```python
from build123d import *
from OCP.BRepFilletAPI import BRepFilletAPI_MakeChamfer

# Parameters (mm, degrees)
SKETCH1_W           = 8
SKETCH1_H           = 7
BOSS_EXTRUDE1_DEPTH = 17
BOSS_EXTRUDE2_DEPTH = 4
CHAMFER1_SIZE       = 2.5
CHAMFER1_SIZE_2     = 2
SKETCH3_R           = 0.4
CUT_EXTRUDE1_DEPTH  = 18.811513131
FILLET2_R           = 0.5
SKETCH4_W           = 0.5
SKETCH4_H           = 15.4
CUT_EXTRUDE2_DEPTH  = 19.814887722
SKETCH5_W           = 0.3
SKETCH5_H           = 11.5
CUT_EXTRUDE3_DEPTH  = 19.814887722
SKETCH6_R           = 0.9
CUT_EXTRUDE4_DEPTH  = 18
CHAMFER2_SIZE       = 0.5
BOSS_EXTRUDE3_START = 2
SKETCH7_R           = 2.5
SKETCH7_R_2         = 0.9
BOSS_EXTRUDE3_DEPTH = 2
BOSS_EXTRUDE4_START = 1.5
SKETCH8_R           = 0.9
SKETCH8_R_2         = 1
BOSS_EXTRUDE4_DEPTH = 1.5
BOSS_EXTRUDE5_START = 1.4
SKETCH9_R           = 1.25
SKETCH9_R_2         = 0.9
BOSS_EXTRUDE5_DEPTH = 1.4
BOSS_EXTRUDE6_START = 15
SKETCH10_R          = 2
SKETCH10_R_2        = 0.9
BOSS_EXTRUDE6_DEPTH = 15
FILLET3_R           = 0.2


# Some blends are built 0.0001 mm under size
with BuildPart() as part:
    # Sketch1 → Boss-Extrude1 (new body)
    with BuildSketch(Plane(origin=(0, 0, 0), x_dir=(1, 0, 0), z_dir=(0, 1, 0))):
        Rectangle(SKETCH1_W, SKETCH1_H)
    extrude(amount=BOSS_EXTRUDE1_DEPTH)

    # Sketch2 → Boss-Extrude2 (add)
    with BuildSketch(Plane(origin=(0, 0, 0), x_dir=(-1, 0, 0), z_dir=(0, -1, 0))):
        Polygon((-2.309401077, 0), (-1.154700538, -2), (1.154700538, -2), (2.309401077, 0), (1.154700538, 2), (-1.154700538, 2), align=None)
    extrude(amount=BOSS_EXTRUDE2_DEPTH)

    # Chamfer1
    chamfer1_edges_1 = [part.edges().sort_by_distance(p)[0] for p in [
        (1.732050808, -4, -1),
    ]]
    chamfer1_side_1 = [part.faces().sort_by_distance(p)[0] for p in [
        (1.732050808, -3.96, -1),
    ]]
    chamfer1_edges_2 = [part.edges().sort_by_distance(p)[0] for p in [
        (1.732050808, -4, 1),
    ]]
    chamfer1_side_2 = [part.faces().sort_by_distance(p)[0] for p in [
        (1.732050808, -3.96, 1),
    ]]
    chamfer1_edges_3 = [part.edges().sort_by_distance(p)[0] for p in [
        (0, -4, 2),
    ]]
    chamfer1_side_3 = [part.faces().sort_by_distance(p)[0] for p in [
        (0, -3.96, 2),
    ]]
    chamfer1_edges_4 = [part.edges().sort_by_distance(p)[0] for p in [
        (-1.732050808, -4, 1),
    ]]
    chamfer1_side_4 = [part.faces().sort_by_distance(p)[0] for p in [
        (-1.732050808, -3.96, 1),
    ]]
    chamfer1_edges_5 = [part.edges().sort_by_distance(p)[0] for p in [
        (-1.732050808, -4, -1),
    ]]
    chamfer1_side_5 = [part.faces().sort_by_distance(p)[0] for p in [
        (-1.732050808, -3.96, -1),
    ]]
    chamfer1_edges_6 = [part.edges().sort_by_distance(p)[0] for p in [
        (0, -4, -2),
    ]]
    chamfer1_side_6 = [part.faces().sort_by_distance(p)[0] for p in [
        (0, -3.96, -2),
    ]]
    chamfer1 = BRepFilletAPI_MakeChamfer(part.part.solid().wrapped)
    for e in chamfer1_edges_1:
        chamfer1.Add(CHAMFER1_SIZE - 0.0001, CHAMFER1_SIZE_2 - 0.0001, e.wrapped, chamfer1_side_1[0].wrapped)
    for e in chamfer1_edges_2:
        chamfer1.Add(CHAMFER1_SIZE - 0.0001, CHAMFER1_SIZE_2 - 0.0001, e.wrapped, chamfer1_side_2[0].wrapped)
    for e in chamfer1_edges_3:
        chamfer1.Add(CHAMFER1_SIZE - 0.0001, CHAMFER1_SIZE_2 - 0.0001, e.wrapped, chamfer1_side_3[0].wrapped)
    for e in chamfer1_edges_4:
        chamfer1.Add(CHAMFER1_SIZE - 0.0001, CHAMFER1_SIZE_2 - 0.0001, e.wrapped, chamfer1_side_4[0].wrapped)
    for e in chamfer1_edges_5:
        chamfer1.Add(CHAMFER1_SIZE - 0.0001, CHAMFER1_SIZE_2 - 0.0001, e.wrapped, chamfer1_side_5[0].wrapped)
    for e in chamfer1_edges_6:
        chamfer1.Add(CHAMFER1_SIZE - 0.0001, CHAMFER1_SIZE_2 - 0.0001, e.wrapped, chamfer1_side_6[0].wrapped)
    add(Compound.cast(chamfer1.Shape()), mode=Mode.REPLACE)  # a hair under: the kernel refuses the full size

    # Sketch3 → Cut-Extrude1 (cut, through all)
    with BuildSketch(Plane(origin=(0, 0, 0), x_dir=(-1, 0, 0), z_dir=(0, -1, 0))):
        with Locations(Location((0, 0, 0), (0, 0, 300))):
            Circle(SKETCH3_R)
    extrude(amount=CUT_EXTRUDE1_DEPTH, mode=Mode.SUBTRACT)

    # Fillet2
    # the kernel refuses this fillet: 0.5 mm, written as the material it takes off along each edge
    with BuildSketch(Plane(origin=(1.334556511, -1.110696502, -2.311519683), x_dir=(0.65389042348858, 0.264929316245572, 0.7086887691106577), z_dir=(-0.3392737411625274, -0.7345565425685966, 0.5876393573674692)), Plane(origin=(-1.334556511, -1.110696502, -2.311519683), x_dir=(0.940687689170844, 0.2649293162455729, -0.2119413334771459), z_dir=(0.33927374116252723, -0.7345565425685966, 0.5876393573674691)), Plane(origin=(2.669113022, -1.110696502, 0), x_dir=(-0.2867972656822634, 0.26492931624557164, 0.9206301025878043), z_dir=(-0.6785474823250541, -0.7345565425685965, 0)), Plane(origin=(-2.669113022, -1.110696502, 0), x_dir=(0.2867972656822621, 0.2649293162455703, -0.9206301025878052), z_dir=(0.6785474823250541, -0.7345565425685966, 0))) as fillet2_piece_1:
        with BuildLine():
            CenterArc((FILLET2_R * 0.424096417587, FILLET2_R), FILLET2_R, 224.036746285, 45.963253715)
            Line((-FILLET2_R * 0.294797720102, FILLET2_R * 0.304880428418), (0, 0))
            Line((0, 0), (FILLET2_R * 0.424096417587, 0))
        make_face()
    extrude(amount=3.874194565, mode=Mode.SUBTRACT)
    with BuildSketch(Plane(origin=(1.334556511, -1.110696502, 2.311519683), x_dir=(0.6538904234885794, 0.26492931624557287, -0.708688769110658), z_dir=(-0.33927374116252706, -0.7345565425685967, -0.5876393573674692)), Plane(origin=(-1.334556511, -1.110696502, 2.311519683), x_dir=(0.9406876891708441, 0.2649293162455719, 0.2119413334771472), z_dir=(0.33927374116252734, -0.7345565425685966, -0.5876393573674692))) as fillet2_piece_2:
        with BuildLine():
            CenterArc((FILLET2_R * 0.424096417587, -FILLET2_R), FILLET2_R, 90, 45.963253715)
            Line((-FILLET2_R * 0.294797720102, -FILLET2_R * 0.304880428418), (0, 0))
            Line((0, 0), (FILLET2_R * 0.424096417587, 0))
        make_face()
    extrude(amount=3.874194565, mode=Mode.SUBTRACT)

    # Sketch4 → Cut-Extrude2 (cut, through all)
    with BuildSketch(Plane.XY.offset(3.5)):
        with Locations((-3.75, 8.5)):
            Rectangle(SKETCH4_W, SKETCH4_H)
    extrude(amount=-CUT_EXTRUDE2_DEPTH, mode=Mode.SUBTRACT)

    # Sketch5 → Cut-Extrude3 (cut, through all)
    with BuildSketch(Plane.XY.offset(3.5)):
        with Locations((3.85, 5.75)):
            Rectangle(SKETCH5_W, SKETCH5_H)
    extrude(amount=-CUT_EXTRUDE3_DEPTH, mode=Mode.SUBTRACT)

    # Sketch6 → Cut-Extrude4 (cut)
    with BuildSketch(Plane(origin=(0, 17, 0), x_dir=(1, 0, 0), z_dir=(0, 1, 0))):
        with Locations(Location((0, 0, 0), (0, 0, 270))):
            Circle(SKETCH6_R)
    extrude(amount=-CUT_EXTRUDE4_DEPTH, mode=Mode.SUBTRACT)

    # Chamfer2
    chamfer2_edges = [part.edges().sort_by_distance(p)[0] for p in [
        (0, -1, -0.9),
    ]]
    chamfer(chamfer2_edges, length=CHAMFER2_SIZE - 0.0001)  # a hair under: the kernel refuses the full size

    # Sketch7 → Boss-Extrude3 (add)
    with BuildSketch(Plane(origin=(0, 17, 0), x_dir=(1, 0, 0), z_dir=(0, 1, 0)).offset(BOSS_EXTRUDE3_START)):
        with Locations(Location((0, 0, 0), (0, 0, 270))):
            Circle(SKETCH7_R)
        with Locations(Location((0, 0, 0), (0, 0, 270))):
            Circle(SKETCH7_R_2, mode=Mode.SUBTRACT)
    extrude(amount=-BOSS_EXTRUDE3_DEPTH)

    # Sketch8 → Boss-Extrude4 (add)
    with BuildSketch(Plane(origin=(0, 19, 0), x_dir=(1, 0, 0), z_dir=(0, 1, 0)).offset(BOSS_EXTRUDE4_START)):
        with BuildLine():
            Line((2.0625, 3.572354791), (5.8125, 1.407291281))
            ThreePointArc((5.8125, 1.407291281), (6.625, 0), (5.8125, -1.407291281))
            Line((5.8125, -1.407291281), (2.0625, -3.572354791))
            ThreePointArc((2.0625, -3.572354791), (0, -4.125), (-2.0625, -3.572354791))
            Line((-2.0625, -3.572354791), (-5.8125, -1.407291281))
            ThreePointArc((-5.8125, -1.407291281), (-6.625, 0), (-5.8125, 1.407291281))
            Line((-5.8125, 1.407291281), (-2.0625, 3.572354791))
            ThreePointArc((-2.0625, 3.572354791), (0, 4.125), (2.0625, 3.572354791))
        make_face()
        with Locations(Location((0, 0, 0), (0, 0, 270))):
            Circle(SKETCH8_R, mode=Mode.SUBTRACT)
        with Locations(Location((5, 0, 0), (0, 0, 270))):
            Circle(SKETCH8_R_2, mode=Mode.SUBTRACT)
        with Locations(Location((-5, 0, 0), (0, 0, 270))):
            Circle(SKETCH8_R_2, mode=Mode.SUBTRACT)
    extrude(amount=-BOSS_EXTRUDE4_DEPTH)

    # Sketch9 → Boss-Extrude5 (add)
    with BuildSketch(Plane(origin=(0, 20.5, 0), x_dir=(1, 0, 0), z_dir=(0, 1, 0)).offset(BOSS_EXTRUDE5_START)):
        with Locations(Location((0, 0, 0), (0, 0, 270))):
            Circle(SKETCH9_R)
        with Locations(Location((0, 0, 0), (0, 0, 270))):
            Circle(SKETCH9_R_2, mode=Mode.SUBTRACT)
    extrude(amount=-BOSS_EXTRUDE5_DEPTH)

    # Sketch10 → Boss-Extrude6 (add)
    with BuildSketch(Plane(origin=(0, 21.9, 0), x_dir=(1, 0, 0), z_dir=(0, 1, 0)).offset(BOSS_EXTRUDE6_START)):
        with Locations(Location((0, 0, 0), (0, 0, 270))):
            Circle(SKETCH10_R)
        with Locations(Location((0, 0, 0), (0, 0, 270))):
            Circle(SKETCH10_R_2, mode=Mode.SUBTRACT)
    extrude(amount=-BOSS_EXTRUDE6_DEPTH)

    # Fillet3
    fillet3_edges = [part.edges().sort_by_distance(p)[0] for p in [
        (6.625, 20.5, 0),
        (3.9375, 20.5, -2.489823036),
        (0, 20.5, -4.125),
        (-3.9375, 20.5, -2.489823036),
        (-6.625, 20.5, 0),
        (-3.9375, 20.5, 2.489823036),
        (0, 20.5, 4.125),
        (3.9375, 20.5, 2.489823036),
        (6.625, 19, 0),
        (3.9375, 19, -2.489823036),
        (0, 19, -4.125),
        (-3.9375, 19, -2.489823036),
        (-6.625, 19, 0),
        (-3.9375, 19, 2.489823036),
        (0, 19, 4.125),
        (3.9375, 19, 2.489823036),
        (0, 36.9, -2),
        (0, 21.9, -2),
    ]]
    fillet(fillet3_edges, radius=FILLET3_R)


solid = part.part
```
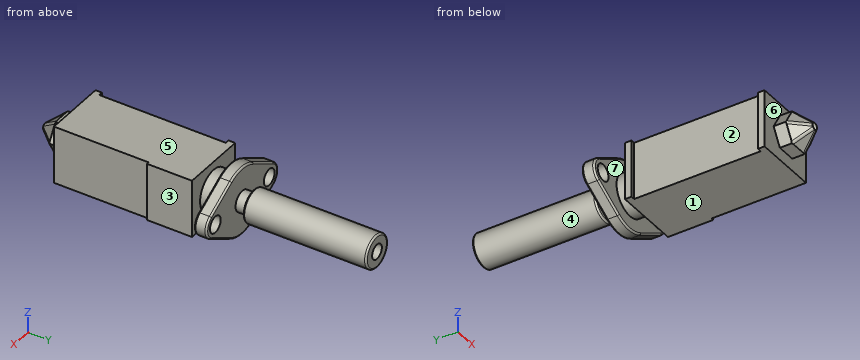
Model file for the job. Use its own axes, mm. Face numbers are marked on the shaded views. A direction names the side the tool comes from. Coordinates: 2 decimals unless noted, no trailing zeros. Order: outer loops, then holes, each group sorted by start corner. A loop starts at its lowest first (then second) coordinate and runs counter-clockwise, first axis right, second up. Notation, with made-up numbers: (44, 77) -> (103, 77) arc R5 cw to (103, 82) -> close; hole circle Ø11 at (54.25, 58). An arc over 180 degrees is marked (long way). Return JSON: item names as keys, results as strings.
Item 1: 3-axis set-ups, long thin cutter, end or side, ignore diameter. For the marked faces 1, 2, 3 and 4: which of +Z, -Z, +X, -X, +Y, -Y reach the whole face in a straight line?
Model answer:
{"face 1": "-Z, +X, -X, -Y", "face 2": "+Z, -Z, -X", "face 3": "+Z, -Z, +X, -Y", "face 4": "+Y"}
Item 2: Pin check, flat tips, straight feed: P1, Ø2, axis at y = 19.5, z = -2, coming from the +X side; P2, Ø1, axis at x = -3, y = 12, coming from the -Z side; P3, Ø3, axis at x = -5, z = 0, coming from the -Y side; P4, Ø1.8, axis at x = 5, z = 0, coming from the +Y side. Stop position of each tip, or through.
Model answer:
{"P1": "stops at x = 6.28", "P2": "stops at z = -3.5", "P3": "stops at y = 0", "P4": "passes through"}
Item 3: Mould opens along Y. For the marked faces 5, 6 and 7 say: pulls with the +Y half, pulls with the -Y half, needs draft (parallel to the pull), parting line crosses it, or undercut.
Model answer:
{"face 5": "needs draft", "face 6": "pulls with the -Y half", "face 7": "undercut"}
Item 4: Wall check: line 1 along Y through (x, z) = (3, 0); line 2 along X through (y, z) = (32, 0); line 3 along Y through (x, z) = (-2, 1.25). Give the ranges that are in metal, low to high. Write a range as from..to.
Model answer:
{"line 1": "y = 0..17, 19..20.5", "line 2": "x = -2..-0.9, 0.9..2", "line 3": "y = 0..20.5"}
Item 5: Slice it at B-B (y = 25). Write the cut outline in (x, z).
Model answer:
{"outline": "circle Ø4 at (0, 0); hole circle Ø1.8 at (0, 0)"}
Item 6: Slice it at A-A (y = 5). Write the cut outline in (x, z).
Model answer:
{"outline": "(-3.5, -3.5) -> (3.7, -3.5) -> (3.7, 3.5) -> (-3.5, 3.5) -> close; hole circle Ø1.8 at (0, 0)"}
